For this review, take the finished solid that the model builds, in its own axes (mm). A direction names the side the tool comes from. Give positions to 0.01 mm unless a question says otherwise; leave off trailing zeros. Write each loop counter-clockwise with the first axis right and the second up, starting at its lowest first coordinate (ties: lowest second). Pieces come first, ordered by that corner, then holes.
1) We need section A-A on z = 34. Give the boundary of the cut face in (x, y).
2) Wall thickness on line 1 along Z through (x, y) = (13, 6); line 2 along X through (y, z) = (-3.5, 122); line 3 along X through (y, z) = (-5, 35): over which ranges is each line inside the solid? List them lowest first.
3) Machinability: for faces 1 (the face through (3.934, -3.356, 75.471)), 2 (the face through (1.23, 4.96, 75.47)), 3 (the face through (1.922, -4.738, 75.471)), 4 (the face through (-1.21, 5.03, 75.47)), 5 (the face through (-5.3, 0.51, 75.47)), which of the approach directions +Z, -Z, +X, -X, +Y, -Y give a long, thin tool a straight path to every point of the face, cutting with its end or side? Answer none if there is none.
4) For P1, Ø8, axis at x = -4, z = 85, coming from the -Y side; P2, Ø12, axis at y = 2, z = 116, coming from the +X side; P3, Ø4, axis at x = 0, z = 34.5, coming from the -Y side, all flat-tipped, find the tip position at first contact; note any pin that passes through.
from build123d import *

# Parameters (mm, degrees)
F1_DEPTH = 150
F2_R     = 0.5
F3_R     = 17.5
F4_DEPTH = 3
F5_R     = 2


with BuildPart() as f1:
    # F0 (on Top) → F1 (new body)
    with BuildSketch(Plane.XY):
        Polygon((3.178624, -1.032797), (8.321745, 2.703899), (1.964497, 2.703899), (0, 8.75), (-1.964497, 2.703899), (-8.321745, 2.703899), (-3.178624, -1.032797), (-5.143121, -7.078899), (0, -3.342203), (5.143121, -7.078899), align=None)
    extrude(amount=F1_DEPTH)

    # F2
    f2_edges = [f1.edges().sort_by_distance(p)[0] for p in [
        (-8.321745, 2.703899, 75),
        (-3.178624, -1.032797, 75),
        (5.143121, -7.078899, 75),
        (0, 8.75, 75),
        (8.321745, 2.703899, 75),
    ]]
    fillet(f2_edges, radius=F2_R)

    # F3 (on Top) → F4 (join)
    with BuildSketch(Plane.XY):
        Circle(F3_R)
    extrude(amount=F4_DEPTH)

    # F5
    f5_edges = [f1.edges().sort_by_distance(p)[0] for p in [
        (-17.5, 0, 3),
    ]]
    fillet(f5_edges, radius=F5_R)


solid = f1.part
Results list:
1. outline: (-7.08, 1.8) - (-3.47, -0.82) arc R0.5 cw to (-3.29, -1.38) - (-5.14, -7.08) - (0, -3.34) - (3.9, -6.17) arc R0.5 ccw to (4.67, -5.62) - (3.18, -1.03) - (7.08, 1.8) arc R0.5 ccw to (6.78, 2.7) - (1.96, 2.7) - (0.48, 7.29) arc R0.5 ccw to (-0.48, 7.29) - (-1.96, 2.7) - (-6.78, 2.7) arc R0.5 ccw to start
2. line 1: z = 0 to 3
2. line 2: x = -3.98 to -0.22, 0.22 to 3.98
2. line 3: x = -4.47 to -2.28, 2.28 to 4.47
3. face 1: +Z, +X
3. face 2: +Z, +X, +Y
3. face 3: +Z, -Y
3. face 4: +Z, -X, +Y
3. face 5: +Z, -X
4. P1: stops at y = -7.08
4. P2: stops at x = 7.28
4. P3: stops at y = -4.8
